Design review of the part built by this model. Coordinates are the model's own, in mm. A direction names the side the tool comes from. Round coordinates to 2 decimals unless told otherwise and drop trailing zeros. Order: outer loops, then holes, each group sorted by start corner. A loop starts at its lowest first (then second) coordinate and runs counter-clockwise, first axis right, second up. Notation, with made-up numbers: M -26.75,-38 L 21.25,-38 A18 cw 21.25,-24 Z; hole C 47,78 d9. An arc over 180 degrees is marked long. Write each question's results on one line, items separated by ' | '. Start each with the question number.
Item 1: Machinability: for faces 1 (the flat face through (-20, -4, 0)), 2 (the cylindrical face through (-19.284, -4.93, -19.253)), which of the approach directions +Z, -Z, +X, -X, +Y, -Y give a long, thin tool a straight path to every point of the face, cutting with its end or side? Answer none if there is none.
Item 2: Wall thickness on line 1 (X direction, y = -9, z = 4); line 2 (X direction, y = -8.5, z = -10.5); line 3 (X direction, y = -5.25, z = 7.5): over which ranges is each line inside the solid? List them lowest first. Write a range as [from, to].
Item 3: Take a section at A-A, the plane z = 5. Write out the cut boundary in (x, y), plus the area to 3 significant figures.
Item 4: Take a section at B-B, the plane y = -8.75. Count the separate pieces of the cut face and the enclosed holes in it, plus the area to 3 significant figures.
Item 5: The part is to be moulded in two halves that separate along Z. For faces 3 (the cylindrical face through (9.925, -4.93, -24.301)), 4 (the cylindrical face through (-27.25, -4.93, 0.02)), 5 (the cylindrical face through (19.253, -4.93, -19.284)), say which applies: +Z half, -Z half, draft (parallel to the pull), parting line (faces both ways), or undercut.
Item 6: Clearance check with flat-ended pins moving along their axes: pin 1 (4 mm diameter, centred on x = 6.5, y = -7.5, fed in from -Z); pin 2 (5 mm diameter, centred on y = -7.5, z = -1.5, fed in from +X); pin 3 (2 mm diameter, centred on x = -16, z = -6, fed in from -Y); pin 4 (3 mm diameter, centred on x = -1, y = 0.5, fed in from -Z). State where each tip first meets the part, or that it passes through.
```python
from build123d import *

# Parameters (mm, degrees)
F0_R     = 26.25
F0_R_2   = 14
F1_DEPTH = 10
F2_R     = 32.5
F2_R_2   = 14
F3_DEPTH = 2
F4_R     = 1
F5_DEPTH = 10
F7_DEPTH = 25


with BuildPart() as f1:
    # F0 (on Front) → F1 (new body)
    with BuildSketch(Plane.XZ):
        Circle(F0_R)
        Circle(F0_R_2, mode=Mode.SUBTRACT)
    extrude(amount=F1_DEPTH)

    # F2 (on Front) → F3 (join)
    with BuildSketch(Plane.XZ):
        Circle(F2_R)
        Circle(F2_R_2, mode=Mode.SUBTRACT)
    extrude(amount=-F3_DEPTH)

    # F4 (on face) → F5 (join, through all)
    with BuildSketch(Plane.XZ):
        with Locations((0, 26.25)):
            Circle(F4_R)
        with Locations((26.25, 0)):
            Circle(F4_R)
        with Locations((0, -26.25)):
            Circle(F4_R)
        with Locations((-26.25, 0)):
            Circle(F4_R)
        with Locations((-18.561553, 18.561553)):
            Circle(F4_R)
        with Locations((-18.561553, -18.561553)):
            Circle(F4_R)
        with Locations((18.561553, -18.561553)):
            Circle(F4_R)
        with Locations((18.561553, 18.561553)):
            Circle(F4_R)
    extrude(amount=F5_DEPTH)

    # F6 (on face) → F7 (cut)
    with BuildSketch(Plane.XZ.offset(10)):
        with BuildLine():
            ThreePointArc((-24.655819, -2.157105), (-23.604495, -7.442469), (-21.434129, -12.375))
            Line((-21.434129, -12.375), (-13.423394, -7.75))
            ThreePointArc((-13.423394, -7.75), (-14.782613, -4.66094), (-15.441018, -1.350914))
            Line((-15.441018, -1.350914), (-24.655819, -2.157105))
        make_face()
        with BuildLine():
            ThreePointArc((-20.274013, -14.196017), (-16.720858, -18.247614), (-12.375, -21.434129))
            Line((-12.375, -21.434129), (-7.75, -13.423394))
            ThreePointArc((-7.75, -13.423394), (-10.471648, -11.427799), (-12.696857, -8.890435))
            Line((-12.696857, -8.890435), (-20.274013, -14.196017))
        make_face()
        with BuildLine():
            ThreePointArc((-10.459802, -22.431118), (-5.35688, -24.163326), (0, -24.75))
            Line((0, -24.75), (0, -15.5))
            ThreePointArc((0, -15.5), (-3.354814, -15.132588), (-6.550583, -14.047771))
            Line((-6.550583, -14.047771), (-10.459802, -22.431118))
        make_face()
        with BuildLine():
            ThreePointArc((2.157105, -24.655819), (7.442469, -23.604495), (12.375, -21.434129))
            Line((12.375, -21.434129), (7.75, -13.423394))
            ThreePointArc((7.75, -13.423394), (4.66094, -14.782613), (1.350914, -15.441018))
            Line((1.350914, -15.441018), (2.157105, -24.655819))
        make_face()
        with BuildLine():
            ThreePointArc((14.196017, -20.274013), (18.247614, -16.720858), (21.434129, -12.375))
            Line((21.434129, -12.375), (13.423394, -7.75))
            ThreePointArc((13.423394, -7.75), (11.427799, -10.471648), (8.890435, -12.696857))
            Line((8.890435, -12.696857), (14.196017, -20.274013))
        make_face()
        with BuildLine():
            ThreePointArc((22.431118, -10.459802), (24.163326, -5.35688), (24.75, 0))
            Line((24.75, 0), (15.5, 0))
            ThreePointArc((15.5, 0), (15.132588, -3.354814), (14.047771, -6.550583))
            Line((14.047771, -6.550583), (22.431118, -10.459802))
        make_face()
        with BuildLine():
            ThreePointArc((24.655819, 2.157105), (23.604495, 7.442469), (21.434129, 12.375))
            Line((21.434129, 12.375), (13.423394, 7.75))
            ThreePointArc((13.423394, 7.75), (14.782613, 4.66094), (15.441018, 1.350914))
            Line((15.441018, 1.350914), (24.655819, 2.157105))
        make_face()
        with BuildLine():
            ThreePointArc((20.274013, 14.196017), (16.720858, 18.247614), (12.375, 21.434129))
            Line((12.375, 21.434129), (7.75, 13.423394))
            ThreePointArc((7.75, 13.423394), (10.471648, 11.427799), (12.696857, 8.890435))
            Line((12.696857, 8.890435), (20.274013, 14.196017))
        make_face()
        with BuildLine():
            ThreePointArc((10.459802, 22.431118), (5.35688, 24.163326), (0, 24.75))
            Line((0, 24.75), (0, 15.5))
            ThreePointArc((0, 15.5), (3.354814, 15.132588), (6.550583, 14.047771))
            Line((6.550583, 14.047771), (10.459802, 22.431118))
        make_face()
        with BuildLine():
            ThreePointArc((-2.157105, 24.655819), (-7.442469, 23.604495), (-12.375, 21.434129))
            Line((-12.375, 21.434129), (-7.75, 13.423394))
            ThreePointArc((-7.75, 13.423394), (-4.66094, 14.782613), (-1.350914, 15.441018))
            Line((-1.350914, 15.441018), (-2.157105, 24.655819))
        make_face()
        with BuildLine():
            ThreePointArc((-14.196017, 20.274013), (-18.247614, 16.720858), (-21.434129, 12.375))
            Line((-21.434129, 12.375), (-13.423394, 7.75))
            ThreePointArc((-13.423394, 7.75), (-11.427799, 10.471648), (-8.890435, 12.696857))
            Line((-8.890435, 12.696857), (-14.196017, 20.274013))
        make_face()
        with BuildLine():
            ThreePointArc((-22.431118, 10.459802), (-24.163326, 5.35688), (-24.75, 0))
            Line((-24.75, 0), (-15.5, 0))
            ThreePointArc((-15.5, 0), (-15.132588, 3.354814), (-14.047771, 6.550583))
            Line((-14.047771, 6.550583), (-22.431118, 10.459802))
        make_face()
    extrude(amount=-F7_DEPTH, mode=Mode.SUBTRACT)


solid = f1.part
```
Results list:
1) face 1: +Y, -Y | face 2: -Y
2) line 1: [-25.94, -24.42], [-14.97, -13.42], [13.42, 14.97], [24.42, 25.94] | line 2: [-24.06, -22.41], [-18.19, -15], [-11.4, -9.26], [9.26, 11.4], [18.19, 24.06] | line 3: [-25.16, -23.59], [-16.08, -11.82], [11.82, 13.56], [23.59, 25.16]
3) outline: M -32.11,0 L -25.77,0 L -25.77,-10 L -24.24,-10 L -24.24,2 L -32.11,2 Z; M -14.67,-10 L -13.08,-10 L -13.08,2 L -14.67,2 Z; M 13.08,-10 L 14.67,-10 L 14.67,2 L 13.08,2 Z; M 24.24,-10 L 25.77,-10 L 25.77,0 L 32.11,0 L 32.11,2 L 24.24,2 Z | area: 100 mm²
4) separate pieces: 1 | enclosed holes: 13 | area: 587 mm²
5) face 3: -Z half | face 4: parting line | face 5: undercut
6) pin 1: z = -25.86 | pin 2: x = 27.25 | pin 3: through | pin 4: z = -32.5
